```python
from build123d import *

# Parameters (mm, degrees)
F2_SIZE  = 0.3
F3_R     = 1.5
F4_DEPTH = 25


with BuildPart() as f1:
    # F0 (on Front) → F1 (revolve)
    with BuildSketch(Plane.XZ):
        Polygon((-5, 0), (-4, 0), (-4, 15), (-5, 15), (-5, 5), (-11, 5), (-11, 1.5), (-5, 1.5), align=None)
    revolve(axis=Axis((0, 0, -3.111579), (0, 0, -1)))

    # F2
    f2_edges = [f1.edges().sort_by_distance(p)[0] for p in [
        (11, 0, 5),
        (5, 0, 15),
        (11, 0, 1.5),
        (5, 0, 0),
    ]]
    chamfer(f2_edges, length=F2_SIZE)

    # F3 (on face) → F4 (cut)
    with BuildSketch(Plane.XY.offset(5)):
        with Locations((0, 8)):
            Circle(F3_R)
        with Locations((-8, 0)):
            Circle(F3_R)
        with Locations((0, -8)):
            Circle(F3_R)
        with Locations((8, 0)):
            Circle(F3_R)
    extrude(amount=-F4_DEPTH, mode=Mode.SUBTRACT)


solid = f1.part
```
Geometry check sheet. Reference: the model listing, model coordinates, mm. A direction names the side the tool comes from. Give positions to 0.01 mm unless a question says otherwise; leave off trailing zeros. Write each loop counter-clockwise with the first axis right and the second up, starting at its lowest first coordinate (ties: lowest second). Pieces come first, ordered by that corner, then holes. Notation, with made-up numbers: (-18, 30) - (12, 30) arc R20 ccw to (12, 45) - close; hole circle Ø7 at (5, -10.75). An arc over 180 degrees is marked (long way). Use a Markdown table: item, result.
Q1. Set-up check for faces 5 (the face through (-2, -5, 1.5)), 6 (the face through (2.38, -10.74, 3.23)), 7 (the face through (1.08, -4.88, 9.78)): record each of +Z, -Z, +X, -X, +Y, -Y from which the full face is reachable in a straight line by a thin tool's end or side.
Computed:
| item | result |
|---|---|
| face 5 | -Z |
| face 6 | +Z, -Z |
| face 7 | +Z |
Q2. Draft check along X on faces 1 (the face through (-9.5, 0.07, 3.27)), 2 (the face through (1.08, -4.88, 0.89)), 3 (the face through (-0.325, 6.536, 3.274)), 4 (the face through (2, -5, 5)). Enter one of: pulls with the +X half, pulls with the -X half, needs draft (parallel to the pull), parting line crosses it, or undercut.
Computed:
| item | result |
|---|---|
| face 1 | undercut |
| face 2 | parting line crosses it |
| face 3 | undercut |
| face 4 | needs draft |
Q3. Section check B-B, the plane z = 12.75. Enter the section's corners in (x, y).
Computed:
| item | result |
|---|---|
| outline | circle Ø10 at (0, 0); hole circle Ø8 at (0, 0) |
Q4. Section check A-A, the plane x = 0. Give the number of separate pieces and of enclosed holes in the cut face, then the cut area to 3 significant figures.
Computed:
| item | result |
|---|---|
| separate pieces | 4 |
| enclosed holes | 0 |
| area | 50.6 mm² |
Q5. Go/stop test with flat-tipped pins: P1, Ø6.5, axis at x = 0, y = 0, coming from the -Z side; P2, Ø4, axis at y = 1.5, z = 13.5, coming from the +X side; P3, Ø6, axis at x = 8, z = 2.5, coming from the -Y side; P4, Ø1, axis at y = 5, z = 13, coming from the -X side. Record where each tip stops, or that it passes through.
Computed:
| item | result |
|---|---|
| P1 | passes through |
| P2 | stops at x = 5 |
| P3 | stops at y = -9.8 |
| P4 | stops at x = -2.18 |
Q6. Thickness scan on L1, parallel to Y at x = 0, z = 2.9; L2, parallel to X at y = -1.25, z = 2.5; L3, parallel to Z at x = 8, y = -3. Record the ranges inside material, lowest first. Write a range as [from, to].
Computed:
| item | result |
|---|---|
| L1 | y = [-11, -9.5], [-6.5, -4], [4, 6.5], [9.5, 11] |
| L2 | x = [-10.93, -8.83], [-7.17, -3.8], [3.8, 7.17], [8.83, 10.93] |
| L3 | z = [1.5, 5] |
